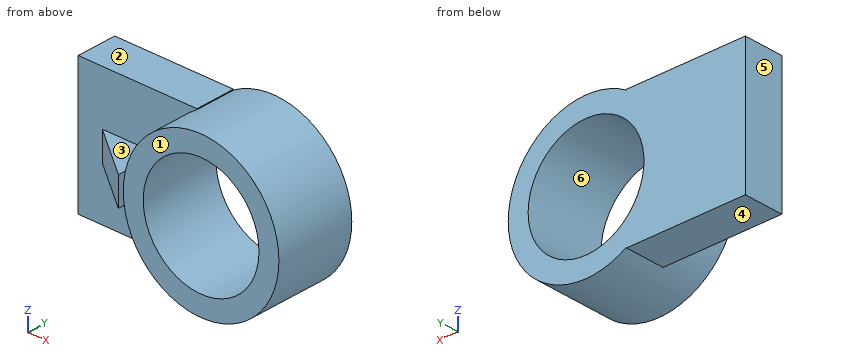
```python
from build123d import *

# Parameters (mm, degrees)
F0_W          = 75.738184
F0_H          = 85.667274
F2_DEPTH      = 25.4
F1_R          = 49.61766
F3_DEPTH      = 50.8
F4_R          = 36.918928
F5_DEPTH      = 50.801
F7_DEPTH      = 8.89
F7_DEPTH_BACK = 9.398


with BuildPart() as f2:
    # F0 (on Front) → F2 (new body)
    with BuildSketch(Plane.XZ):
        with Locations((-38.330909, 0)):
            Rectangle(F0_W, F0_H)
    extrude(amount=F2_DEPTH)

    # F1 (on Front) → F3 (join)
    with BuildSketch(Plane.XZ):
        with Locations((25.399998, 0)):
            Circle(F1_R)
    extrude(amount=F3_DEPTH)

    # F4 (on face) → F5 (cut, through all)
    with BuildSketch(Plane.XZ.offset(50.8)):
        with Locations((25.399998, 0)):
            Circle(F4_R)
    extrude(amount=-F5_DEPTH, mode=Mode.SUBTRACT)

    # F6 (on Top) → F7 (join, two sides)
    with BuildSketch(Plane.XY) as f7_sk:
        Polygon((-61.508864, -24.901086), (-25.902238, -52.381378), (-24.69754, -24.901086), align=None)
    extrude(amount=F7_DEPTH)
    extrude(f7_sk.sketch, amount=-F7_DEPTH_BACK)


solid = f2.part
```
Geometry check sheet. Reference: the model listing, model coordinates, mm. Face numbers are marked on the shaded views. A direction names the side the tool comes from. Coordinates: 2 decimals unless noted, no trailing zeros. Order: outer loops, then holes, each group sorted by start corner. A loop starts at its lowest first (then second) coordinate and runs counter-clockwise, first axis right, second up. Notation, with made-up numbers: M -28.5,55 L -22.5,55 A19 ccw -22.5,80 Z; hole C 73,12.25 d6. An arc over 180 degrees is marked long. Answer as a JSON object with one key per item and string values.
Q1. Release check for a two-part mould opening along X. For the marked faces 4, 5 and 6 record: released by +X, released by -X, zero draft, split by the parting line, or undercut.
Results are:
{"face 4": "zero draft", "face 5": "released by -X", "face 6": "undercut"}
Q2. Tool access check on the marked faces 1, 2 and 3. Record the directions out of +Z, -Z, +X, -X, +Y, -Y that give a thin tool (end or side, any length) a straight path to the whole face; none if there is none.
Results are:
{"face 1": "+Z, -Z, +X, -Y", "face 2": "+Z, -X, +Y, -Y", "face 3": "+Z, -X, -Y"}
Q3. Cross-section at D-D on x = -34.5. Record the cut outline in (y, z).
Results are:
{"outline": "M -45.75,-9.4 L -25.4,-9.4 L -25.4,-42.83 L 0,-42.83 L 0,42.83 L -25.4,42.83 L -25.4,8.89 L -45.75,8.89 Z"}
Q4. Cross-section at B-B on y = -44. Record the cut outline in (x, z), and give its area (3 significant figures).
Results are:
{"outline": "M -36.76,-9.4 L -25.53,-9.4 L -25.53,8.89 L -36.76,8.89 Z; C 25.4,0 d99.24; hole C 25.4,0 d73.84", "area": "3,660 mm²"}
Q5. Cross-section at A-A on z = 0. Record the cut outline in (x, y), and give its area (3 significant figures).
Results are:
{"outline": "M -76.2,-25.4 L -60.86,-25.4 L -25.9,-52.38 L -24.72,-25.4 L -24.22,-25.4 L -24.22,-50.8 L -11.52,-50.8 L -11.52,0 L -76.2,0 Z; M 62.32,-50.8 L 75.02,-50.8 L 75.02,0 L 62.32,0 Z", "area": "3,100 mm²"}
Q6. Depth check by flat-ended pin: pin 1 Ø6 at (y, z) = (-28.5, -5.5) entering from -X; pin 2 Ø8 at (x, y) = (58.5, -5.5) entering from -Z; pin 3 Ø7.5 at (x, y) = (-56.5, -13) entering from +Z. Enter the tip coordinate at first touch or a pass-through.
Results are:
{"pin 1": "stops at x = -60.73", "pin 2": "stops at z = -40.19", "pin 3": "stops at z = 42.83"}
Q7. Cross-section at C-C on x = 41.5. Record the cut outline in (y, z), and give its area (3 significant figures).
Results are:
{"outline": "M -50.8,-46.93 L 0,-46.93 L 0,-33.22 L -50.8,-33.22 Z; M -50.8,33.22 L 0,33.22 L 0,46.93 L -50.8,46.93 Z", "area": "1,390 mm²"}
Q8. Scan lines: line 1 (X direction, y = -34, z = -6.5); line 2 (Y direction, x = -20.5, z = 35.5); line 3 (X direction, y = -10, z = -33). Record each from-to range of solid material in increasing order.
Results are:
{"line 1": "x = -49.72 to -25.1, -23.79 to -10.94, 61.74 to 74.59", "line 2": "y = -25.4 to 0", "line 3": "x = -76.2 to 8.85, 41.95 to 62.45"}
